from build123d import *

# Parameters (mm, degrees)
SKETCH_1_R      = 3.5
SKETCH_1_R_2    = 2.5
EXTRUDE_1_DEPTH = 90
SKETCH_2_R      = 6
SKETCH_2_R_2    = 2.5
EXTRUDE_2_DEPTH = 1
EXTRUDE_START   = -1
SKETCH_3_R      = 6
SKETCH_3_R_2    = 2.5
EXTRUDE_3_DEPTH = 1
FILLET_1_R      = 0.5


with BuildPart() as part:
    # 草图1 → 凸台-拉伸1 (new body)
    with BuildSketch(Plane.XY):
        with Locations(Location((0, 0, 0), (0, 0, 180))):
            Circle(SKETCH_1_R)
        with Locations(Location((0, 0, 0), (0, 0, 180))):
            Circle(SKETCH_1_R_2, mode=Mode.SUBTRACT)
    extrude(amount=EXTRUDE_1_DEPTH)

    # 草图2 → 凸台-拉伸2 (add)
    with BuildSketch(Plane(origin=(0, 0, 0), x_dir=(-1, 0, 0), z_dir=(0, 0, -1))):
        Circle(SKETCH_2_R)
        Circle(SKETCH_2_R_2, mode=Mode.SUBTRACT)
    extrude(amount=-EXTRUDE_2_DEPTH)

    # 草图3 → 凸台-拉伸3 (add)
    with BuildSketch(Plane.XY.offset(90).offset(EXTRUDE_START)):
        with Locations(Location((0, 0, 0), (0, 0, 180))):
            Circle(SKETCH_3_R)
        with Locations(Location((0, 0, 0), (0, 0, 180))):
            Circle(SKETCH_3_R_2, mode=Mode.SUBTRACT)
    extrude(amount=EXTRUDE_3_DEPTH)

    # 圆角1
    fillet_1_edges = [part.edges().sort_by_distance(p)[0] for p in [
        (3.5, 0, 1),
        (6, 0, 1),
        (3.5, 0, 89),
        (6, 0, 89),
    ]]
    fillet(fillet_1_edges, radius=FILLET_1_R)


solid = part.part
Source: CAD feature listing. Evaluate the final solid. Frame: model axes, mm. A direction names the side the tool comes from. Round coordinates to 2 decimals unless told otherwise and drop trailing zeros. Loops run counter-clockwise (first coordinate to the right, second up) from the corner with the lowest first, then second, coordinate; pieces in that order, holes last. Notation, with made-up numbers: (65, -11.75) - (124, -11.75) arc R13 cw to (124, 0.25) - close; hole circle Ø5 at (30.5, 72.25). An arc over 180 degrees is marked (long way). Write item = value, one per line. Start each with the question number.
(1) Ray query, line 1 along Z through (x, y) = (3.25, -2.75); line 2 along Y through (x, z) = (0, 65); line 3 along Y through (x, z) = (-1.5, 6.5). Return the intervals inside material, ascending. Write a range as from..to.
(2) Pull-direction query (Y, two-part tool) for faces 1 (the face through (5.994, 0.264, 0.246)), 2 (the face through (4, -2, 1)), 3 (the face through (2.5, -0.1, 44.4)); classes: +Y half, -Y half, draft (parallel to the pull), parting line (faces both ways), or undercut.
(3) Pin query (flat end, axial travel): pin 1 (1 mm diameter, centred on y = -2, z = 58, fed in from -X); pin 2 (1.5 mm diameter, centred on x = -2, z = 23.5, fed in from -Y); pin 3 (2 mm diameter, centred on x = -1, y = -0.5, fed in from +Z). Return the tip coordinate at first contact, or that it passes through.
(4) Section query A-A, the plane x = 0. Output: boundary loops of the cut face in (y, z), plus the area to 3 significant figures.
(5) Set-up query: faces 4 (the face through (-5.723, -1.802, 89.746)), 5 (the face through (-3.233, 1.341, 44.391)). Return all of +Z, -Z, +X, -X, +Y, -Y with unobstructed straight access to the full face (end or side cutting, diameter ignored); none if empty.
(6) Section query C-C, the plane z = 45. Output: boundary loops of the cut face in (x, y).
Conclusion:
q1.line_1 = 0..1, 89..90
q1.line_2 = -3.5..-2.5, 2.5..3.5
q1.line_3 = -3.16..-2, 2..3.16
q2.face_1 = parting line
q2.face_2 = draft
q2.face_3 = undercut
q3.pin_1 = -3.16
q3.pin_2 = -3.27
q3.pin_3 = through
q4.outline = (-6, 0) - (-2.5, 0) - (-2.5, 90) - (-6, 90) - (-6, 89.5) arc R0.5 ccw to (-5.5, 89) - (-4, 89) arc R0.5 cw to (-3.5, 88.5) - (-3.5, 1.5) arc R0.5 cw to (-4, 1) - (-5.5, 1) arc R0.5 ccw to (-6, 0.5) - close; (2.5, 0) - (6, 0) - (6, 0.5) arc R0.5 ccw to (5.5, 1) - (4, 1) arc R0.5 cw to (3.5, 1.5) - (3.5, 88.5) arc R0.5 cw to (4, 89) - (5.5, 89) arc R0.5 ccw to (6, 89.5) - (6, 90) - (2.5, 90) - close
q4.area = 190 mm2
q5.face_4 = +Z, -Z
q5.face_5 = none
q6.outline = circle Ø7 at (0, 0); hole circle Ø5 at (0, 0)
